Verification items for the finished model (mm, model axes). A direction names the side the tool comes from. Give positions to 0.01 mm unless a question says otherwise; leave off trailing zeros. Write each loop counter-clockwise with the first axis right and the second up, starting at its lowest first coordinate (ties: lowest second). Pieces come first, ordered by that corner, then holes. Notation, with made-up numbers: M -6.5,-29 L 17.5,-29 A13 ccw 17.5,-19 Z; hole C 25,49 d8. An arc over 180 degrees is marked long. Answer as a JSON object with one key per item and string values.
```python
from build123d import *

# Parameters (mm, degrees)
SKETCH1_W           = 270
SKETCH1_H           = 150
BOSS_EXTRUDE2_DEPTH = 5
SKETCH4_W           = 260
SKETCH4_H           = 140
SKETCH4_W_2         = 250
SKETCH4_H_2         = 130
BOSS_EXTRUDE3_DEPTH = 5
FILLET1_R           = 5


with BuildPart() as part:
    # Sketch1 → Boss-Extrude2 (new body)
    with BuildSketch(Plane(origin=(0, 0, 0), x_dir=(1, 0, 0), z_dir=(0, 1, 0))):
        Rectangle(SKETCH1_W, SKETCH1_H)
    extrude(amount=BOSS_EXTRUDE2_DEPTH)

    # Sketch4 → Boss-Extrude3 (add)
    with BuildSketch(Plane(origin=(0, 5, 0), x_dir=(1, 0, 0), z_dir=(0, 1, 0))):
        Rectangle(SKETCH4_W, SKETCH4_H)
        Rectangle(SKETCH4_W_2, SKETCH4_H_2, mode=Mode.SUBTRACT)
    extrude(amount=BOSS_EXTRUDE3_DEPTH)

    # Fillet1
    fillet1_edges = [part.edges().sort_by_distance(p)[0] for p in [
        (-130, 7.5, 70),
        (130, 7.5, 70),
        (130, 7.5, -70),
        (-130, 7.5, -70),
        (-125, 7.5, -65),
        (-125, 7.5, 65),
        (125, 7.5, 65),
        (125, 7.5, -65),
        (0, 0, 75),
        (-135, 0, 0),
        (0, 0, -75),
        (135, 0, 0),
        (135, 2.5, 75),
        (-135, 2.5, 75),
        (-135, 2.5, -75),
        (135, 2.5, -75),
    ]]
    fillet(fillet1_edges, radius=FILLET1_R - 0.0001)  # a hair under: the kernel refuses the full size


solid = part.part
```
1) Thickness scan on L1, parallel to X at y = 5.5, z = 27; L2, parallel to Z at x = -43.5, y = 7; L3, parallel to Y at x = 56.5, z = 6. Record the ranges inside material, lowest first.
Completed:
{"L1": "x = -130 to -125, 125 to 130", "L2": "z = -70 to -65, 65 to 70", "L3": "y = 0 to 5"}
2) Access from +Z, -Z, +X, -X, +Y, -Y to the whole of each face (thin tool, end or side, straight path). Record for faces 1 (the face through (128, 8, 69)), 2 (the face through (2, 2, 74)), 3 (the face through (-2, 5, -1)).
Completed:
{"face 1": "+Z, +X, +Y", "face 2": "+Z, +X, -X, -Y", "face 3": "+Y"}
3) Go/stop test with flat-tipped pins: pin 1 (3 mm diameter, centred on x = -69.5, y = 8, fed in from -Z); pin 2 (4 mm diameter, centred on x = 23, y = 8, fed in from +Z); pin 3 (2 mm diameter, centred on x = -104, y = 3, fed in from +Z). Record where each tip stops, or that it passes through.
Completed:
{"pin 1": "stops at z = -70", "pin 2": "stops at z = 70", "pin 3": "stops at z = 74.9"}
4) Release check for a two-part mould opening along Z. For faces 4 (the face through (124, 8, -63)), 5 (the face through (125, 7, 1)), 6 (the face through (-2, 7, 70)), 7 (the face through (-128, 8, -69)) record: pulls with the +Z half, pulls with the -Z half, needs draft (parallel to the pull), parting line crosses it, or undercut.
Completed:
{"face 4": "undercut", "face 5": "undercut", "face 6": "pulls with the +Z half", "face 7": "pulls with the -Z half"}
5) Section check A-A on y = 7.5. Record the boundary of the cut face in (x, z).
Completed:
{"outline": "M -130,-65 A5 ccw -125,-70 L 125,-70 A5 ccw 130,-65 L 130,65 A5 ccw 125,70 L -125,70 A5 ccw -130,65 Z; hole M -125,-60 A5 ccw -120,-65 L 120,-65 A5 ccw 125,-60 L 125,60 A5 ccw 120,65 L -120,65 A5 ccw -125,60 Z"}
